The model under review builds one solid part; all positions refer to its coordinate system, in mm. A direction names the side the tool comes from. Give positions to 0.01 mm unless a question says otherwise; leave off trailing zeros. Write each loop counter-clockwise with the first axis right and the second up, starting at its lowest first coordinate (ties: lowest second). Pieces come first, ordered by that corner, then holes. Notation, with made-up numbers: M 41.25,58.25 L 49.25,58.25 A28 cw 49.25,83.25 Z; hole C 14,1.5 d4. An arc over 180 degrees is marked long. Write item = value, one per line. Start each with the question number.
```python
from build123d import *

# Parameters (mm, degrees)
F0_W     = 101.6
F0_H     = 101.6
F1_DEPTH = 101.6
F2_R     = 7.011592
F3_DEPTH = 101.6
F4_W     = 50.8
F4_H     = 50.8
F5_DEPTH = 50.8


with BuildPart() as f1:
    # F0 (on Front) → F1 (new body)
    with BuildSketch(Plane.XZ):
        with Locations((-50.8, 50.8)):
            Rectangle(F0_W, F0_H)
    extrude(amount=F1_DEPTH)

    # F2 (on face) → F3 (cut)
    with BuildSketch(Plane.XY.offset(101.6)):
        with Locations((-92.807561, -8.640565)):
            Circle(F2_R)
    extrude(amount=-F3_DEPTH, mode=Mode.SUBTRACT)

    # F4 (on face) → F5 (cut)
    with BuildSketch(Plane.XY.offset(101.6)):
        with Locations((-25.4, -76.2)):
            Rectangle(F4_W, F4_H)
    extrude(amount=-F5_DEPTH, mode=Mode.SUBTRACT)


solid = f1.part
```
Item 1: For faces 1 (the flat face through (-26, -50.8, 77)), 2 (the flat face through (-63, -39, 101.6)), list the 3-axis set-ups (+Z, -Z, +X, -X, +Y, -Y) from which the entire face can be reached by the end or side of a thin tool; tool diameter is ignored.
Item 2: We need section A-A, the plane z = 81.5. Write out the cut boundary in (x, y).
Item 3: Clearance check with flat-ended pins moving along their axes: P1, Ø16, axis at x = -92.81, y = -8.64, coming from the -Z side; P2, Ø15, axis at x = -17, z = 72.5, coming from the -Y side. State where each tip first meets the part, or that it passes through.
Item 4: We need section D-D, the plane x = -89.5. Write out the cut boundary in (y, z).
Item 5: The part is to be moulded in two halves that separate along X. For faces 3 (the flat face through (-101.6, -50, 50)), 4 (the cylindrical face through (-86.12, -6.53, 51.51)), 5 (the flat face through (-52, -50, 0)), 6 (the flat face through (0, -39, 39)), say which applies: released by +X, released by -X, zero draft, split by the parting line, or undercut.
Item 6: We need section C-C, the plane y = -12.5. Write out the cut boundary in (x, z), and give its area (3 significant figures).
Item 7: To check wall thickness, follow probe 1 along X at (y, z) = (-9, 60); probe 2 along X at (y, z) = (-72, 58); probe 3 along Z at (x, y) = (-25.5, -92.5). State the ranges of each line that lie inside material, in increasing order. Write a range as [from, to].
Item 8: We need section B-B, the plane x = -27. Write out the cut boundary in (y, z).
Worked out:
q1.face_1 = +Z, +X, -Y
q1.face_2 = +Z, +X, -X, +Y, -Y
q2.outline = M -101.6,-101.6 L -50.8,-101.6 L -50.8,-50.8 L 0,-50.8 L 0,0 L -101.6,0 Z; hole C -92.81,-8.64 d14.02
q3.P1 = 0
q3.P2 = -50.8
q4.outline = M -101.6,0 L -14.82,0 L -14.82,101.6 L -101.6,101.6 Z; M -2.46,0 L 0,0 L 0,101.6 L -2.46,101.6 Z
q5.face_3 = released by -X
q5.face_4 = undercut
q5.face_5 = zero draft
q5.face_6 = released by +X
q6.outline = M -101.6,0 L -98.66,0 L -98.66,101.6 L -101.6,101.6 Z; M -86.95,0 L 0,0 L 0,101.6 L -86.95,101.6 Z
q6.area = 9,130 mm²
q7.probe_1 = [-101.6, -99.81], [-85.81, 0]
q7.probe_2 = [-101.6, -50.8]
q7.probe_3 = [0, 50.8]
q8.outline = M -101.6,0 L 0,0 L 0,101.6 L -50.8,101.6 L -50.8,50.8 L -101.6,50.8 Z
